Can you work these out from the model? Positions are in its coordinate system, mm. Round coordinates to 2 decimals unless told otherwise and drop trailing zeros. Loops run counter-clockwise (first coordinate to the right, second up) from the corner with the lowest first, then second, coordinate; pieces in that order, holes last.
(1) Will these pins go through, and if not, where does the flat tip stop? pin 1 Ø1.5 at (x, y) = (25, -18) entering from -Z; pin 2 Ø12 at (y, z) = (-15.5, 22.5) entering from -X; pin 3 Ø12 at (x, y) = (14.5, -11.5) entering from -Z; pin 4 Ø3 at (x, y) = (18, -20.5) entering from +Z.
(2) If I drill on line 1 along Z through (x, y) = (29.7, 0); line 2 along Z through (x, y) = (14, 30); line 3 along Y through (x, z) = (18.5, -25), over which ranges is the centre line in solid material (lowest first)?
(3) I want a section at C-C on x = 13.5. Write out the boundary of the cut face in (y, z), plus the area to 3 significant figures.
(4) I want a section at A-A on y = 0. Write out the boundary of the cut face in (x, z), plus the area to 3 significant figures.
(5) Thinking about a two-plate mould opening in Y: for faces 1 (the face through (1.66, -7.45, -33.57)), 2 (the face through (15.28, -8.67, 39.05)), 3 (the face through (31, 18, 30)), which applies, released by +Y, released by -Y, zero draft, split by the parting line, or undercut?
(6) I want a section at D-D on x = 25. Write out the boundary of the cut face in (y, z), plus the area to 3 significant figures.
Autodesk Inventor part; units mm, degrees
ref_plane "IP_1_XY" through (0, 0, 0) normal (1, 0, 0) x (0, 0, -1)
ref_plane "IP_1_YZ" through (0, 0, 0) normal (0, 0, -1) x (0, 1, 0)
ref_plane "IP_1_ZX" through (0, 0, 0) normal (0, 1, 0) x (1, 0, 0)
sketch "Sketch_1" plane through (0, 0, 0) normal (0, 0, 1) x (1, 0, 0)
  line L0 (50, 0) -> (-50, 0)
  line L1 (0, 34.3864) -> (3.2698, 34.3864)
  arc A0 (3.2698, 34.3864) -> (4.1774, 34.6401) centre (3.2698, 36.1364) ccw
  arc A1 (11.3226, 34.6401) -> (4.1774, 34.6401) centre (7.75, 28.75) ccw
  arc A2 (11.3226, 34.6401) -> (12.2302, 34.3864) centre (12.2302, 36.1364) ccw
  line L2 (12.2302, 34.3864) -> (18.7698, 34.3864)
  arc A3 (18.7698, 34.3864) -> (19.6774, 34.6401) centre (18.7698, 36.1364) ccw
  arc A4 (26.8226, 34.6401) -> (19.6774, 34.6401) centre (23.25, 28.75) ccw
  arc A5 (26.8226, 34.6401) -> (27.7302, 34.3864) centre (27.7302, 36.1364) ccw
  line L3 (27.7302, 34.3864) -> (31, 34.3864)
  line L4 (31, 34.3864) -> (31, 40)
  line L5 (31, 40) -> (0, 40)
  line L6 (0, 40) -> (0, 34.3864)
revolve "Revolution1" add sketch "Sketch_1" angle 360 about axis through (50, 0, 0) along (1, 0, 0)
ref_plane "IP_1_XY" through (0, 0, 0) normal (1, 0, 0) x (0, 0, -1)
ref_plane "IP_1_YZ" through (0, 0, 0) normal (0, 0, -1) x (0, 1, 0)
ref_plane "IP_1_ZX" through (0, 0, 0) normal (0, 1, 0) x (1, 0, 0)
ref_plane "IP_2_XY" through (15.5, 0, 0) normal (1, 0, 0) x (0, 0, -1)
ref_plane "IP_2_YZ" through (15.5, 0, 0) normal (0, 0, -1) x (0, 1, 0)
ref_plane "IP_2_ZX" through (15.5, 0, 0) normal (0, 1, 0) x (1, 0, 0)
properties part number "hpc_Q2307-ACC_1"
Filled sheet:
1. pin 1: stops at z = -36.09
1. pin 2: passes through
1. pin 3: stops at z = -39.62
1. pin 4: stops at z = 35.2
2. line 1: z = -40 to -34.39, 34.39 to 40
2. line 2: z = -26.46 to -16.81, 16.81 to 26.46
2. line 3: y = -31.22 to -23.61, 23.61 to 31.22
3. outline: circle Ø80 at (0, 0); hole circle Ø68.77 at (0, 0)
3. area: 1,310 mm2
4. outline: (0, -40) - (31, -40) - (31, -34.39) - (27.73, -34.39) arc R1.75 ccw to (26.82, -34.64) arc R6.89 cw to (19.68, -34.64) arc R1.75 ccw to (18.77, -34.39) - (12.23, -34.39) arc R1.75 ccw to (11.32, -34.64) arc R6.89 cw to (4.18, -34.64) arc R1.75 ccw to (3.27, -34.39) - (0, -34.39) - close; (0, 34.39) - (3.27, 34.39) arc R1.75 ccw to (4.18, 34.64) arc R6.89 cw to (11.32, 34.64) arc R1.75 ccw to (12.23, 34.39) - (18.77, 34.39) arc R1.75 ccw to (19.68, 34.64) arc R6.89 cw to (26.82, 34.64) arc R1.75 ccw to (27.73, 34.39) - (31, 34.39) - (31, 40) - (0, 40) - close
4. area: 321 mm2
5. face 1: undercut
5. face 2: split by the parting line
5. face 3: zero draft
6. outline: circle Ø80 at (0, 0); hole circle Ø70.83 at (0, 0)
6. area: 1,090 mm2
